```python
from build123d import *

# Parameters (mm, degrees)
SKETCH1_R           = 1
SKETCH1_R_2         = 2.3
BOSS_EXTRUDE1_DEPTH = 3
SKETCH2_R           = 0.5
SKETCH2_R_2         = 1
CUT_EXTRUDE1_DEPTH  = 73.097156671


with BuildPart() as part:
    # Sketch1 → Boss-Extrude1 (new body)
    with BuildSketch(Plane(origin=(0, 0, 0), x_dir=(0, 0, -1), z_dir=(1, 0, 0))):
        with BuildLine():
            Line((-5.5, 0), (5.5, 0))
            ThreePointArc((5.5, 0), (7.621320344, 0.878679656), (8.5, 3))
            Line((8.5, 3), (8.5, 67))
            ThreePointArc((8.5, 67), (7.621320344, 69.121320344), (5.5, 70))
            Line((5.5, 70), (-5.5, 70))
            ThreePointArc((-5.5, 70), (-7.621320344, 69.121320344), (-8.5, 67))
            Line((-8.5, 67), (-8.5, 3))
            ThreePointArc((-8.5, 3), (-7.621320344, 0.878679656), (-5.5, 0))
        make_face()
        with Locations((0, 3.35)):
            Circle(SKETCH1_R, mode=Mode.SUBTRACT)
        with Locations(Location((0, 30.65, 0), (0, 0, 180))):
            Circle(SKETCH1_R, mode=Mode.SUBTRACT)
        with Locations(Location((0, 53, 0), (0, 0, 180))):
            Circle(SKETCH1_R_2, mode=Mode.SUBTRACT)
        with BuildLine():
            Line((-6.5, 27.75), (-6.5, 6.25))
            ThreePointArc((-6.5, 6.25), (-6.207106781, 5.542893219), (-5.5, 5.25))
            Line((-5.5, 5.25), (5.5, 5.25))
            ThreePointArc((5.5, 5.25), (6.207106781, 5.542893219), (6.5, 6.25))
            Line((6.5, 6.25), (6.5, 27.75))
            ThreePointArc((6.5, 27.75), (6.207106781, 28.457106781), (5.5, 28.75))
            Line((5.5, 28.75), (-5.5, 28.75))
            ThreePointArc((-5.5, 28.75), (-6.207106781, 28.457106781), (-6.5, 27.75))
        make_face(mode=Mode.SUBTRACT)
    extrude(amount=BOSS_EXTRUDE1_DEPTH)

    # Sketch2 → Cut-Extrude1 (cut, through all)
    with BuildSketch(Plane(origin=(0, 0, -8.5), x_dir=(-1, 0, 0), z_dir=(0, 0, -1))):
        with Locations((-1.5, 58)):
            Circle(SKETCH2_R)
        with Locations(Location((-1.5, 48, 0), (0, 0, 180))):
            Circle(SKETCH2_R)
        with Locations((-1.5, 53)):
            Circle(SKETCH2_R_2)
    extrude(amount=-CUT_EXTRUDE1_DEPTH, mode=Mode.SUBTRACT)


solid = part.part
```
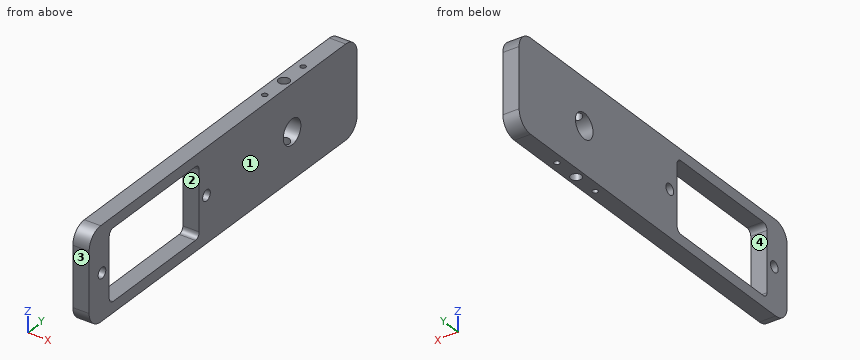
For this review, take the finished solid that the model builds, in its own axes (mm). Face numbers are marked on the shaded views. Coordinates: 2 decimals unless noted, no trailing zeros. Loops run counter-clockwise (first coordinate to the right, second up) from the corner with the lowest first, then second, coordinate; pieces in that order, holes last. Notation, with made-up numbers: (29, 39) -> (48, 39) arc R26 ccw to (48, 54) -> close; hole circle Ø4 at (-6.75, 51). An arc over 180 degrees is marked (long way). Return JSON: item names as keys, results as strings. Group by question number.
(1) To check wall thickness, follow L1, parallel to Y at x = 1.5, z = 4.25; L2, parallel to X at y = 58, z = -2.75; L3, parallel to X at y = 53, z = -5. State the ranges of each line that lie inside material, in increasing order.
(2) Consider section C-C, the plane y = 18. Give the boundary of the cut face in (x, z).
(3) Consider section B-B, the plane y = 30.65. Give the boundary of the cut face in (x, z), plus the area to 3 significant figures.
(4) Mouldability with a two-part tool opening along Y and no side actions: class the marked faces 1, 2, 3 and 4 as pulls with the +Y half, pulls with the -Y half, needs draft (parallel to the pull), parting line crosses it, or undercut.
(5) Consider section A-A, the plane x = 1.5. Count the separate pieces of the cut face and the enclosed holes in it, plus the area to 3 significant figures.
Results below:
{
 "1": {"L1": "y = 0 to 5.25, 28.75 to 47.5, 48.5 to 52, 54 to 57.5, 58.5 to 70", "L2": "x = 0 to 1, 2 to 3", "L3": "x = 0 to 0.5, 2.5 to 3"},
 "2": {"outline": "(0, -8.5) -> (3, -8.5) -> (3, -6.5) -> (0, -6.5) -> close; (0, 6.5) -> (3, 6.5) -> (3, 8.5) -> (0, 8.5) -> close"},
 "3": {"outline": "(0, -8.5) -> (3, -8.5) -> (3, -1) -> (0, -1) -> close; (0, 1) -> (3, 1) -> (3, 8.5) -> (0, 8.5) -> close", "area": "45.0 mm2"},
 "4": {"face 1": "needs draft", "face 2": "undercut", "face 3": "pulls with the -Y half", "face 4": "undercut"},
 "5": {"separate pieces": "4", "enclosed holes": "3", "area": "796 mm2"}
}
